Source: three-view drawing plus pictorial views. Frame: mm from the lowest corner of the part. A direction names the side the tool comes from. Coordinates: 2 decimals unless noted, no trailing zeros. Loops run counter-clockwise (first coordinate to the right, second up) from the corner with the lowest first, then second, coordinate; pieces in that order, holes last. Notation, with made-up numbers: (-38.5, -26) -> (14.5, -26) arc R26 ccw to (14.5, 0) -> close; hole circle Ø11 at (15, 84). An arc over 180 degrees is marked (long way). Answer as a JSON object with one key per item and string values. Group by question number.
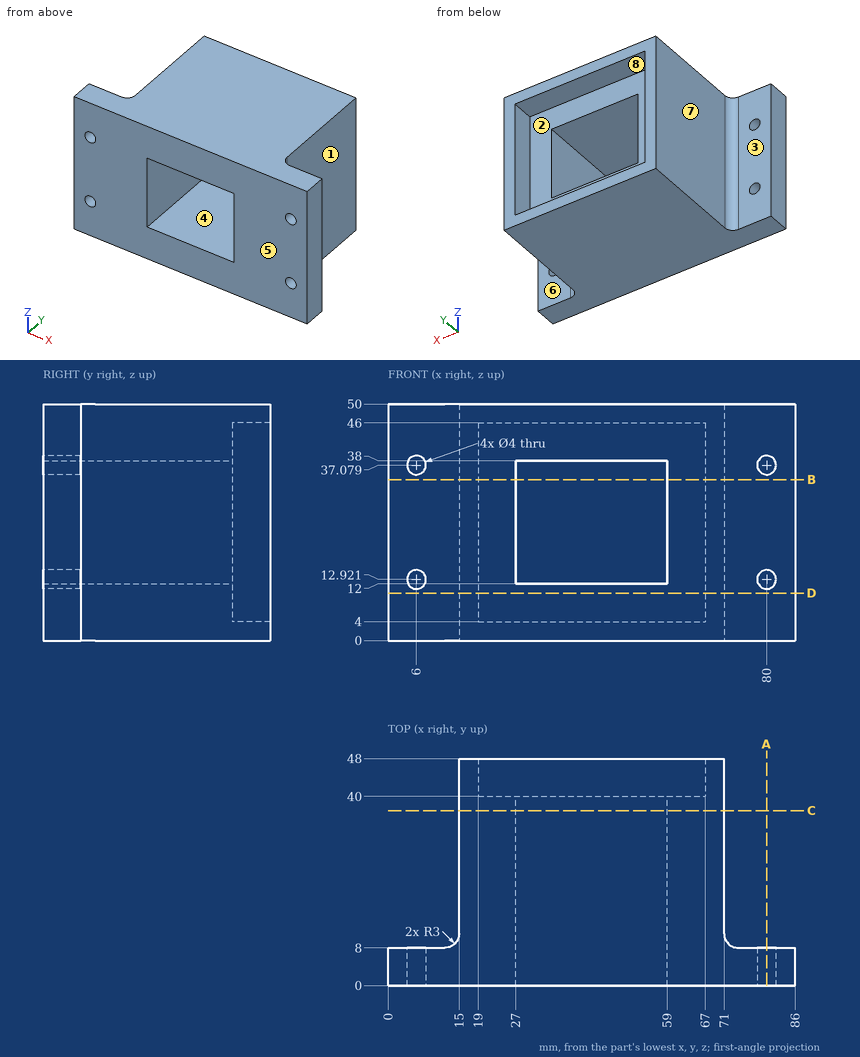
1. Reachability of the marked faces 4, 5, 6, 7 and 8 from +Z, -Z, +X, -X, +Y, -Y: full face, straight path, thin tool, end or side. Return the list, or none.
2. Section query C-C on y = 37. Return loops of the section in (x, z).
3. Section query D-D on z = 10. Return loops of the section in (x, y).
4. Section query A-A on x = 80. Return loops of the section in (y, z).
5. Mould query, pull axis X, two halves, no side actions, for the marked faces 1, 2 and 3. Classes: pulls with the +X half, pulls with the -X half, needs draft (parallel to the pull), parting line crosses it, or undercut.
6. Pin query (flat end, axial travel): pin 1 Ø6 at (x, z) = (77, 17.5) entering from +Y; pin 2 Ø6.5 at (y, z) = (43.5, 26.5) entering from +X; pin 3 Ø2 at (y, z) = (13.5, 27) entering from -X. Return the tip coordinate at first contact, or that it passes through.
7. Ray query, L1, parallel to Z at x = 80, y = 2; L2, parallel to X at y = 22, z = 21.5; L3, parallel to X at y = 40.5, z = 5.5. Return the intervals inside material, ascending.
8. Section query B-B on z = 34. Return loops of the section in (x, y).
Solved:
{
 "1": {"face 4": "+Y, -Y", "face 5": "+Z, -Z, +X, -X, -Y", "face 6": "+Z, -Z, +X, +Y", "face 7": "+Z, -Z, -X, +Y", "face 8": "+Y"},
 "2": {"outline": "(15, 0) -> (71, 0) -> (71, 50) -> (15, 50) -> close; hole (27, 12) -> (59, 12) -> (59, 38) -> (27, 38) -> close"},
 "3": {"outline": "(0, 0) -> (86, 0) -> (86, 8) -> (74, 8) arc R3 cw to (71, 11) -> (71, 48) -> (67, 48) -> (67, 40) -> (19, 40) -> (19, 48) -> (15, 48) -> (15, 11) arc R3 cw to (12, 8) -> (0, 8) -> close"},
 "4": {"outline": "(0, 0) -> (8, 0) -> (8, 10.92) -> (0, 10.92) -> close; (0, 14.92) -> (8, 14.92) -> (8, 35.08) -> (0, 35.08) -> close; (0, 39.08) -> (8, 39.08) -> (8, 50) -> (0, 50) -> close"},
 "5": {"face 1": "pulls with the +X half", "face 2": "undercut", "face 3": "needs draft"},
 "6": {"pin 1": "y = 8", "pin 2": "x = 71", "pin 3": "x = 15"},
 "7": {"L1": "0 to 10.92, 14.92 to 35.08, 39.08 to 50", "L2": "15 to 27, 59 to 71", "L3": "15 to 19, 67 to 71"},
 "8": {"outline": "(0, 0) -> (27, 0) -> (27, 40) -> (19, 40) -> (19, 48) -> (15, 48) -> (15, 11) arc R3 cw to (12, 8) -> (0, 8) -> close; (59, 0) -> (86, 0) -> (86, 8) -> (74, 8) arc R3 cw to (71, 11) -> (71, 48) -> (67, 48) -> (67, 40) -> (59, 40) -> close"}
}
